Input: dimensioned drawing with shaded views. Units: mm. Origin: part minimum x, y, z. A direction names the side the tool comes from. Round coordinates to 2 decimals unless told otherwise and drop trailing zeros. Write each loop counter-clockwise with the first axis right and the second up, starting at its lowest first coordinate (ties: lowest second). Pieces come first, ordered by that corner, then holes. Notation, with made-up numbers: (-3, 81) -> (43, 81) arc R27 cw to (43, 120) -> close; hole circle Ø3 at (8.5, 47). An arc over 180 degrees is marked (long way). Use one line per item in the form item = value. Start each with the question number.
1. Reachability of the marked faces 1, 2 and 3 from +Z, -Z, +X, -X, +Y, -Y: full face, straight path, thin tool, end or side. Return the list, or none.
2. Line query: L1, parallel to Y at x = 3, z = 1.2; L2, parallel to X at y = 2.2, z = 1.25; L3, parallel to Z at x = 2.5, y = 1. Output: solid intervals per line, ascending.
3. Cut plane D-D, the plane z = 12. Return the cut outline in (x, y), plus the area to 3 significant figures.
4. Cut plane A-A, the plane z = 8. Return the cut outline in (x, y).
5. Cut plane B-B, the plane x = 3. Return the cut outline in (y, z).
6. Cut plane C-C, the plane y = 1.15. Return the cut outline in (x, z).
7. Pin query (flat end, axial travel): pin 1 Ø0.5 at (x, y) = (3, 2) entering from -Z. Return the tip coordinate at first contact, or that it passes through.
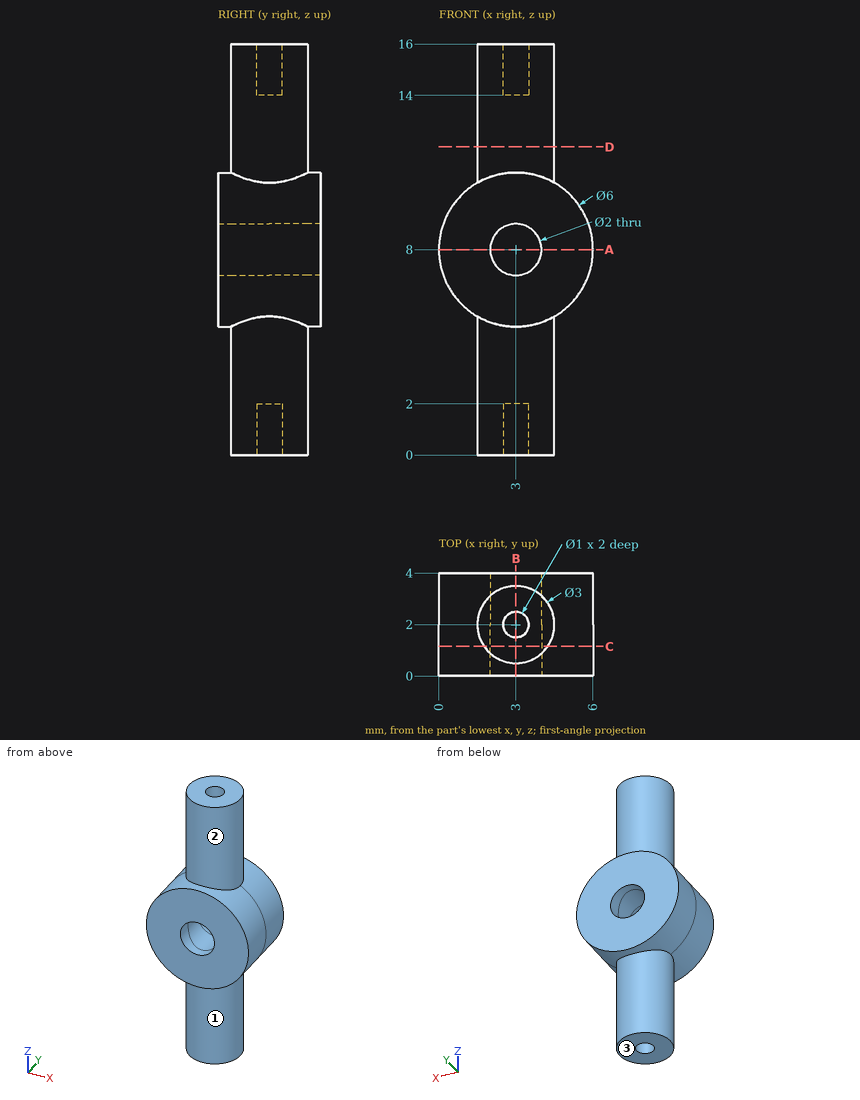
Outcome:
q1.face_1 = -Z
q1.face_2 = +Z
q1.face_3 = -Z, +X, -X, +Y, -Y
q2.L1 = 0.5 to 1.5, 2.5 to 3.5
q2.L2 = 1.51 to 2.54, 3.46 to 4.49
q2.L3 = 0 to 7.13, 8.87 to 16
q3.outline = circle Ø3 at (3, 2)
q3.area = 7.07 mm^2
q4.outline = (0, 0) -> (2, 0) -> (2, 4) -> (0, 4) -> close; (4, 0) -> (6, 0) -> (6, 4) -> (4, 4) -> close
q5.outline = (0, 5) -> (0.5, 5) -> (0.5, 0) -> (1.5, 0) -> (1.5, 2) -> (2.5, 2) -> (2.5, 0) -> (3.5, 0) -> (3.5, 5) -> (4, 5) -> (4, 7) -> (0, 7) -> close; (0, 9) -> (4, 9) -> (4, 11) -> (3.5, 11) -> (3.5, 16) -> (2.5, 16) -> (2.5, 14) -> (1.5, 14) -> (1.5, 16) -> (0.5, 16) -> (0.5, 11) -> (0, 11) -> close
q6.outline = (1.76, 0) -> (4.24, 0) -> (4.24, 5.27) arc R3 ccw to (4.24, 10.73) -> (4.24, 16) -> (1.76, 16) -> (1.76, 10.73) arc R3 ccw to (1.76, 5.27) -> close; hole circle Ø2 at (3, 8)
q7.pin_1 = 2
